Could you check a few things on this model? Use its own coordinates, in mm. A direction names the side the tool comes from. Round coordinates to 2 decimals unless told otherwise and drop trailing zeros. Loops run counter-clockwise (first coordinate to the right, second up) from the corner with the lowest first, then second, coordinate; pieces in that order, holes last. Notation, with made-up numbers: (-11, -11) -> (23, -11) arc R23 ccw to (23, 25) -> close; hole circle Ø10 at (62, -34). An arc over 180 degrees is marked (long way). One line per item, written item: value.
```python
from build123d import *

# Parameters (mm, degrees)
SKIZZE1_R                       = 55.154328933
AUFSATZ_LINEAR_AUSTRAGEN1_DEPTH = 3
SKIZZE1_2_R                     = 58.154328933
SKIZZE1_2_R_2                   = 55.154328933
LINEAR_AUSTRAGEN_D_NN1_DEPTH    = 20
SKIZZE2_W                       = 10
SKIZZE2_H                       = 13.341521541
SKIZZE2_W_2                     = 25.935051322
SKIZZE2_H_2                     = 5
SCHNITT_LINEAR_AUSTRAGEN1_DEPTH = 59.154328933
KREISMUSTER1_COUNT              = 4
SCHNITT_LINEAR_AUSTRAGEN5_REACH = 5
SKIZZE4_R                       = 2.5


with BuildPart() as part:
    # Skizze1 → Aufsatz-Linear austragen1 (new body)
    with BuildSketch(Plane(origin=(0, 0, 0), x_dir=(1, 0, 0), z_dir=(0, 1, 0))):
        Circle(SKIZZE1_R)
    extrude(amount=AUFSATZ_LINEAR_AUSTRAGEN1_DEPTH)

    # Skizze1_2 → Linear-Austragen-D_nn1 (add)
    with BuildSketch(Plane(origin=(0, 0, 0), x_dir=(1, 0, 0), z_dir=(0, 1, 0))):
        Circle(SKIZZE1_2_R)
        Circle(SKIZZE1_2_R_2, mode=Mode.SUBTRACT)
    extrude(amount=LINEAR_AUSTRAGEN_D_NN1_DEPTH)

    # Skizze2 → Schnitt-Linear austragen1 (cut, through all)
    with BuildSketch(Plane(origin=(0, 0, 0), x_dir=(0, 0, -1), z_dir=(1, 0, 0))):
        with Locations((-17.349848993, 13.32923923)):
            Rectangle(SKIZZE2_W, SKIZZE2_H)
        with Locations((0.617676668, 9.158478459)):
            Rectangle(SKIZZE2_W_2, SKIZZE2_H_2)
    schnitt_linear_austragen1 = extrude(amount=-SCHNITT_LINEAR_AUSTRAGEN1_DEPTH, mode=Mode.SUBTRACT)

    # Kreismuster1: Schnitt-Linear austragen1 ×4 about axis
    kreismuster1_axis = Axis((0, 0, 0), (0, 1, 0))
    for i in range(1, KREISMUSTER1_COUNT):
        add(schnitt_linear_austragen1.rotate(kreismuster1_axis, i * 360 / KREISMUSTER1_COUNT), mode=Mode.SUBTRACT)

    # Skizze4 → Schnitt-Linear austragen5 (cut, up to next)
    with BuildSketch(Plane(origin=(0, 3, 0), x_dir=(1, 0, 0), z_dir=(0, 1, 0)), mode=Mode.PRIVATE) as schnitt_linear_austragen5_sk1:
        with Locations((-25, 0)):
            Circle(SKIZZE4_R)
    schnitt_linear_austragen5_tool1 = extrude(schnitt_linear_austragen5_sk1.sketch, amount=-SCHNITT_LINEAR_AUSTRAGEN5_REACH, mode=Mode.PRIVATE) & part.part
    add(schnitt_linear_austragen5_tool1.solids().sort_by_distance((-25, 3, 0))[0], mode=Mode.SUBTRACT)
    # Skizze4 → Schnitt-Linear austragen5 (cut, up to next)
    with BuildSketch(Plane(origin=(0, 3, 0), x_dir=(1, 0, 0), z_dir=(0, 1, 0)), mode=Mode.PRIVATE) as schnitt_linear_austragen5_sk2:
        with Locations((25, 0)):
            Circle(SKIZZE4_R)
    schnitt_linear_austragen5_tool2 = extrude(schnitt_linear_austragen5_sk2.sketch, amount=-SCHNITT_LINEAR_AUSTRAGEN5_REACH, mode=Mode.PRIVATE) & part.part
    add(schnitt_linear_austragen5_tool2.solids().sort_by_distance((25, 3, 0))[0], mode=Mode.SUBTRACT)


solid = part.part
```
(1) Imagine slicing it at B-B on y = 8.25. Write out the boundary of the cut face in (x, z).
Results below:
outline: (-56.55, -13.59) arc R58.15 ccw to (-22.35, -53.69) -> (-22.35, -50.42) arc R55.15 cw to (-53.46, -13.59) -> close; (-53.69, 22.35) -> (-50.42, 22.35) arc R55.15 cw to (-13.59, 53.46) -> (-13.59, 56.55) arc R58.15 ccw to start; (13.59, -56.55) arc R58.15 ccw to (53.69, -22.35) -> (50.42, -22.35) arc R55.15 cw to (13.59, -53.46) -> close; (22.35, 50.42) arc R55.15 cw to (53.46, 13.59) -> (56.55, 13.59) arc R58.15 ccw to (22.35, 53.69) -> close
(2) For pin 1 Ø8 at (x, y) = (44.5, 16) entering from +Z; pin 2 Ø6 at (x, y) = (19.5, 14.5) entering from +Z; pin 3 Ø0.9 at (x, y) = (-55.5, 17) entering from +Z; pin 4 Ø2.5 at (x, z) = (-55, 1) entering from -Y, each with a flat end and sliding along its axis, tell me the tip position at first contact or that it passes through.
Results below:
pin 1: stops at z = 41.73
pin 2: stops at z = 53.69
pin 3: stops at z = 12.35
pin 4: stops at y = 0
(3) Imagine slicing it at D-D on y = 14.75. Write out the boundary of the cut face in (x, z), then the cut area to 3 significant figures.
Results below:
outline: (-56.83, 12.35) arc R58.15 ccw to (-22.35, -53.69) -> (-22.35, -50.42) arc R55.15 cw to (-53.75, 12.35) -> close; (-53.69, 22.35) -> (-50.42, 22.35) arc R55.15 cw to (12.35, 53.75) -> (12.35, 56.83) arc R58.15 ccw to start; (-12.35, -56.83) arc R58.15 ccw to (53.69, -22.35) -> (50.42, -22.35) arc R55.15 cw to (-12.35, -53.75) -> close; (22.35, 50.42) arc R55.15 cw to (53.75, -12.35) -> (56.83, -12.35) arc R58.15 ccw to (22.35, 53.69) -> close
area: 942 mm²
(4) On a 3-axis mill with a long thin cutter (end or side, diameter ignored), from which of +Z, -Z, +X, -X, +Y, -Y can I reach the whole of each face in a straight line? I mean faces 1 (the face through (-5, 6.658, -56)), 2 (the face through (-22.35, 13, -52)), 3 (the face through (-52, 13, 22.35)), 4 (the face through (5, 6.658, 56)). Say none if no direction works.
Results below:
face 1: -Z
face 2: -Z, +Y
face 3: -X, +Y
face 4: +Z
(5) We'd pull the mould along Y, two halves only. Please class faces 5 (the face through (-13.585, 9, 55)), 6 (the face through (22.5, 1.5, -0.1)), 7 (the face through (-26, 20, 49)): +Y half, -Y half, draft (parallel to the pull), parting line (faces both ways), or undercut.
Results below:
face 5: undercut
face 6: draft
face 7: +Y half
(6) Imagine slicing it at A-A on x = 0. Write out the boundary of the cut face in (y, z).
Results below:
outline: (0, -58.15) -> (6.66, -58.15) -> (6.66, -55.15) -> (3, -55.15) -> (3, 55.15) -> (6.66, 55.15) -> (6.66, 58.15) -> (0, 58.15) -> close; (11.66, -58.15) -> (20, -58.15) -> (20, -55.15) -> (11.66, -55.15) -> close; (11.66, 55.15) -> (20, 55.15) -> (20, 58.15) -> (11.66, 58.15) -> close
(7) Imagine slicing it at C-C on x = 25. Write out the boundary of the cut face in (y, z), then the cut area to 3 significant figures.
Results below:
outline: (0, -52.51) -> (20, -52.51) -> (20, -49.16) -> (3, -49.16) -> (3, -2.5) -> (0, -2.5) -> close; (0, 2.5) -> (3, 2.5) -> (3, 49.16) -> (20, 49.16) -> (20, 52.51) -> (0, 52.51) -> close
area: 414 mm²
(8) Please list where these lines run through material, in increasing order: L1, parallel to X at y = 2.35, z = 0; L2, parallel to X at y = 4.5, z = -13.5; L3, parallel to X at y = 13.25, z = 0.
Results below:
L1: x = -58.15 to -27.5, -22.5 to 22.5, 27.5 to 58.15
L2: x = -56.57 to -53.48, 53.48 to 56.57
L3: x = -58.15 to -55.15, 55.15 to 58.15
